Geometry check sheet. Reference: the model listing, model coordinates, mm. Round coordinates to 2 decimals unless told otherwise and drop trailing zeros. Use one line per item in the form item = value.
from build123d import *

# Parameters (mm, degrees)
BOSS_EXTRUDE1_DEPTH = 3.175
SKETCH3_R           = 3.175
CUT_EXTRUDE2_DEPTH  = 219.245167472


with BuildPart() as part:
    # Sketch1 → Boss-Extrude1 (new body)
    with BuildSketch(Plane.XY):
        Polygon((-215.9, 0), (215.9, 0), (215.9, -31.75), (132.08, -31.75), (127, -26.67), (-127, -26.67), (-132.08, -31.75), (-215.9, -31.75), align=None)
    extrude(amount=BOSS_EXTRUDE1_DEPTH)

    # Sketch3 → Cut-Extrude2 (cut, through all)
    with BuildSketch(Plane.XY.offset(3.175)):
        with Locations((-199.39, -15.24)):
            Circle(SKETCH3_R)
        with Locations((-187.96, -15.24)):
            Circle(SKETCH3_R)
        with Locations((-176.53, -15.24)):
            Circle(SKETCH3_R)
        with Locations((-165.1, -15.24)):
            Circle(SKETCH3_R)
        with Locations((-153.67, -15.24)):
            Circle(SKETCH3_R)
        with Locations((-142.24, -15.24)):
            Circle(SKETCH3_R)
        with Locations((-130.81, -15.24)):
            Circle(SKETCH3_R)
        with Locations((-119.38, -15.24)):
            Circle(SKETCH3_R)
        with Locations((-107.95, -15.24)):
            Circle(SKETCH3_R)
        with Locations((-96.52, -15.24)):
            Circle(SKETCH3_R)
        with Locations((-85.09, -15.24)):
            Circle(SKETCH3_R)
        with Locations((-73.66, -15.24)):
            Circle(SKETCH3_R)
        with Locations((-62.23, -15.24)):
            Circle(SKETCH3_R)
        with Locations((-50.8, -15.24)):
            Circle(SKETCH3_R)
        with Locations((-39.37, -15.24)):
            Circle(SKETCH3_R)
        with Locations((-27.94, -15.24)):
            Circle(SKETCH3_R)
        with Locations((-16.51, -15.24)):
            Circle(SKETCH3_R)
        with Locations((-5.08, -15.24)):
            Circle(SKETCH3_R)
        with Locations((6.35, -15.24)):
            Circle(SKETCH3_R)
        with Locations((17.78, -15.24)):
            Circle(SKETCH3_R)
        with Locations((29.21, -15.24)):
            Circle(SKETCH3_R)
        with Locations((40.64, -15.24)):
            Circle(SKETCH3_R)
        with Locations((52.07, -15.24)):
            Circle(SKETCH3_R)
        with Locations((63.5, -15.24)):
            Circle(SKETCH3_R)
        with Locations((74.93, -15.24)):
            Circle(SKETCH3_R)
        with Locations((86.36, -15.24)):
            Circle(SKETCH3_R)
        with Locations((97.79, -15.24)):
            Circle(SKETCH3_R)
        with Locations((109.22, -15.24)):
            Circle(SKETCH3_R)
        with Locations((120.65, -15.24)):
            Circle(SKETCH3_R)
        with Locations((132.08, -15.24)):
            Circle(SKETCH3_R)
        with Locations((143.51, -15.24)):
            Circle(SKETCH3_R)
        with Locations((154.94, -15.24)):
            Circle(SKETCH3_R)
        with Locations((166.37, -15.24)):
            Circle(SKETCH3_R)
        with Locations((177.8, -15.24)):
            Circle(SKETCH3_R)
        with Locations((189.23, -15.24)):
            Circle(SKETCH3_R)
        with Locations((200.66, -15.24)):
            Circle(SKETCH3_R)
    extrude(amount=-CUT_EXTRUDE2_DEPTH, mode=Mode.SUBTRACT)


solid = part.part
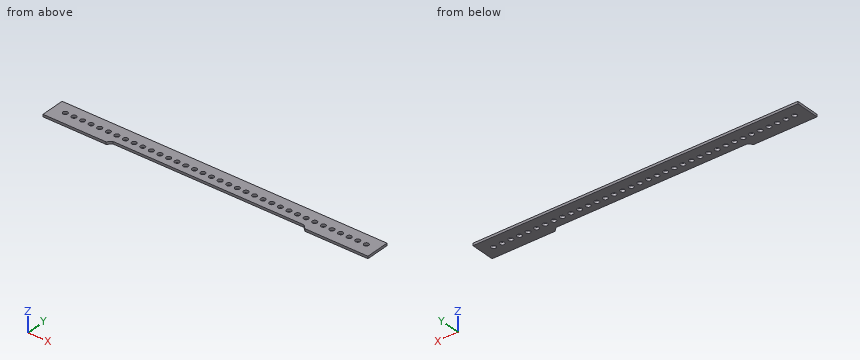
1. Gauge pin test, flat end, axial feed: pin 1 (4 mm diameter, centred on x = 132.08, y = -15.24, fed in from -Z). Record the tip position at first contact, or that the pin passes through.
Return value:
pin_1 = through
2. Section check A-A (z = 1). Count the separate pieces of the cut face and the enclosed holes in it, then the cut area to 3 significant figures.
Return value:
separate_pieces = 1
enclosed_holes = 36
area = 11,300 mm2
3. Material ranges on line 1 along Y through (x, z) = (-142.5, 2.5); line 2 along Y through (x, z) = (-16.51, 1.25) (3 decimals), recorded low to high.
Return value:
line_1 = -31.75 to -18.4, -12.08 to 0
line_2 = -26.67 to -18.415, -12.065 to 0
